Read the model definition and answer for the solid it produces. Units are mm, in the model's axes. Face numbers are marked on the shaded views. A direction names the side the tool comes from. Round coordinates to 2 decimals unless told otherwise and drop trailing zeros. Loops run counter-clockwise (first coordinate to the right, second up) from the corner with the lowest first, then second, coordinate; pieces in that order, holes last. Notation, with made-up numbers: M -21,79.25 L 24,79.25 A19 ccw 24,90.25 Z; hole C 32,19 d8. An arc over 180 degrees is marked long. Write each question's results on one line, items separated by ' | '.
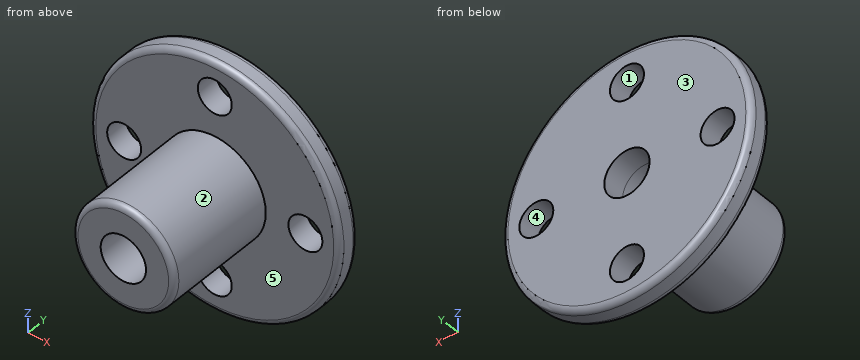
Autodesk Inventor part; units mm, degrees
ref_plane "YZ Plane" through (0, 0, 0) normal (1, 0, 0) x (0, 1, 0)
ref_plane "XZ Plane" through (0, 0, 0) normal (0, 1, 0) x (-1, 0, 0)
ref_plane "XY Plane" through (0, 0, 0) normal (0, 0, 1) x (1, 0, 0)
sketch "Sketch1" plane through (0, 0, 0) normal (0, 1, 0) x (-1, 0, 0)
  circle A0 centre (0, 0) radius 11
  circle A1 centre (0, 0) radius 2
  circle A2 centre (8, 0) radius 1.5
  circle A3 centre (0, 8) radius 1.5
  circle A4 centre (-8, 0) radius 1.5
  circle A5 centre (0, -8) radius 1.5
  dimension "d0" = 22
  dimension "d1" = 4
  dimension "d2" = 3
  dimension "d3" = 8
  dimension "d6" = 360
extrude "Extrusion1" add sketch "Sketch1" along normal blind 2
fillet "Fillet1" radius 0.5 2 edges at (11, 2, 0) (11, 0, 0)
sketch "Sketch2" plane through (0, 0, 0) normal (0, -1, 0) x (1, 0, 0)
  circle A0 centre (0, 0) radius 2
  circle A1 centre (0, 0) radius 4.5
  dimension "d11" = 9
extrude "Extrusion2" add sketch "Sketch2" along normal blind 10
fillet "Fillet2" radius 0.5 1 edges at (-4.5, -10, 0)
properties part number "WH-Coupling-4mm"
Item 1: The part is cut by section C-C (y = -7.75). Determine the outline of the cut face in (x, z), plus the area to 3 significant figures.
Outcome:
outline: C 0,0 d9; hole C 0,0 d4 | area: 51.1 mm2
Item 2: For the marked faces 4 and 5, determine the directions among +Z, -Z, +X, -X, +Y, -Y from which every point of the face is accessible in a straight line to the end or side of a thin tool.
Outcome:
face 4: +Y, -Y | face 5: -Y
Item 3: The part is cut by section A-A (z = 0). Determine the outline of the cut face in (x, y).
Outcome:
outline: M -11,0.5 A0.5 ccw -10.5,0 L -9.5,0 L -9.5,2 L -10.5,2 A0.5 ccw -11,1.5 Z; M -6.5,0 L -4.5,0 L -4.5,-9.5 A0.5 ccw -4,-10 L -2,-10 L -2,2 L -6.5,2 Z; M 2,-10 L 4,-10 A0.5 ccw 4.5,-9.5 L 4.5,0 L 6.5,0 L 6.5,2 L 2,2 Z; M 9.5,0 L 10.5,0 A0.5 ccw 11,0.5 L 11,1.5 A0.5 ccw 10.5,2 L 9.5,2 Z
Item 4: The mould has two halves that part along Z. Classify the marked faces 1, 2 and 3: pulls with the +Z half, pulls with the -Z half, needs draft (parallel to the pull), parting line crosses it, or undercut.
Outcome:
face 1: undercut | face 2: parting line crosses it | face 3: needs draft
Item 5: The part is cut by section B-B (x = 0). Determine the outline of the cut face in (y, z).
Outcome:
outline: M -10,-4 A0.5 ccw -9.5,-4.5 L 0,-4.5 L 0,-6.5 L 2,-6.5 L 2,-2 L -10,-2 Z; M -10,2 L 2,2 L 2,6.5 L 0,6.5 L 0,4.5 L -9.5,4.5 A0.5 ccw -10,4 Z; M 0,-10.5 A0.5 ccw 0.5,-11 L 1.5,-11 A0.5 ccw 2,-10.5 L 2,-9.5 L 0,-9.5 Z; M 0,9.5 L 2,9.5 L 2,10.5 A0.5 ccw 1.5,11 L 0.5,11 A0.5 ccw 0,10.5 Z
Item 6: Straight lines are drawn through the part: line 1 (Z direction, x = 0, y = 1.3); line 2 (Y direction, x = 5.25, z = 0.25); line 3 (Z direction, x = 0, y = -6.75). For each, find the intervals that lie inside material, in ascending order.
Outcome:
line 1: z = -11 to -9.5, -6.5 to -2, 2 to 6.5, 9.5 to 11 | line 2: y = 0 to 2 | line 3: z = -4.5 to -2, 2 to 4.5
Item 7: Flat-ended cylindrical pins translate along their axes: pin 1 (5 mm diameter, centred on y = -2, z = -3, fed in from -X); pin 2 (5 mm diameter, centred on x = -6, z = 5, fed in from -Y); pin 3 (4 mm diameter, centred on y = -1.5, z = -7.5, fed in from +X). Find the tip coordinate at first contact, or state that the pin passes through.
Outcome:
pin 1: stops at x = -10.77 | pin 2: stops at y = 0 | pin 3: stops at x = 8.79
